Geometry check sheet. Reference: the model listing, model coordinates, mm. A direction names the side the tool comes from. Round coordinates to 2 decimals unless told otherwise and drop trailing zeros. Order: outer loops, then holes, each group sorted by start corner. A loop starts at its lowest first (then second) coordinate and runs counter-clockwise, first axis right, second up. Notation, with made-up numbers: (2.5, 25.5) - (20.5, 25.5) arc R30 ccw to (20.5, 49.5) - close; hole circle Ø6 at (62, 33.5). An arc over 180 degrees is marked (long way). One line per question, with ' | ' between items. Start each with the question number.
Q1. Sectioned sample at C-C, the plane z = 1.5. Enter the section's corners in (x, y).
Q2. Mould release check, pull along Z, two halves, no side actions. Record for faces 1 (the face through (13, 3, 3)), 2 (the face through (14, 4.5, -1)), 3 (the face through (4.24, 2.22, -0.13)): +Z half, -Z half, draft (parallel to the pull), parting line (faces both ways), or undercut.
Q3. Tool access check on faces 4 (the face through (14, 3, -1.2)), 5 (the face through (11, 5, 0)), 6 (the face through (10.272, 4.735, 0.929)), 7 (the face through (11, 1, 0)), 8 (the face through (6.5, 5, 2)). Record the directions out of +Z, -Z, +X, -X, +Y, -Y that give a thin tool (end or side, any length) a straight path to the whole face; none if there is none.
Q4. Material ranges on line 1 along X through (y, z) = (3, 2); line 2 along Z through (x, y) = (-3.25, 1.5); line 3 along X through (y, z) = (2.65, 0), recorded low to high.
Q5. Sectioned sample at D-D, the plane z = -0.5. Enter the section's corners in (x, y), then the cut area to 3 significant figures.
Q6. Sectioned sample at A-A, the plane y = 3. Enter the section's corners in (x, z).
Q7. Gauge pin test, flat ends, axial feed: P1, Ø1, axis at x = 14, z = -1, coming from the +Y side; P2, Ø2.5, axis at x = 13.5, y = 3, coming from the -Z side; P3, Ø1.2, axis at y = 5.5, z = 2, coming from the -X side. Record the tip position at first contact, or that the pin passes through.
Q8. Sectioned sample at B-B, the plane x = 10.5. Enter the section's corners in (y, z).
```python
from build123d import *

# Parameters (mm, degrees)
SKETCH_2_W          = 13
SKETCH_2_H          = 10
SKETCH_2_R          = 1
EXTRUDE_1_DEPTH     = 6
EXTRUDE_3_DEPTH     = 10
SKETCH_5_R          = 1.75
CUT_EXTRUDE_1_DEPTH = 20.293781382
SKETCH_6_W          = 13
SKETCH_6_H          = 10
CUT_EXTRUDE_2_DEPTH = 1.5


with BuildPart() as part:
    # 草图2 → 凸台-拉伸1 (new body)
    with BuildSketch(Plane(origin=(0, 0, 0), x_dir=(1, 0, 0), z_dir=(0, 1, 0))):
        Rectangle(SKETCH_2_W, SKETCH_2_H)
        with Locations(Location((-3.25, 0, 0), (0, 0, 270))):
            Circle(SKETCH_2_R, mode=Mode.SUBTRACT)
        with Locations(Location((3.25, 0, 0), (0, 0, 270))):
            Circle(SKETCH_2_R, mode=Mode.SUBTRACT)
    extrude(amount=EXTRUDE_1_DEPTH)

    # 草图4 → 凸台-拉伸3 (add)
    with BuildSketch(Plane(origin=(6.5, 0, 11.5), x_dir=(0, 0, -1), z_dir=(1, 0, 0))):
        Polygon((11.5, 6), (11.5, 4.5), (12.7, 4.5), (12.7, 1.5), (11.5, 1.5), (11.5, 0), (8.5, 0), (8.5, 6), align=None)
    extrude(amount=EXTRUDE_3_DEPTH)

    # 草图5 → 切除-拉伸1 (cut, through all)
    with BuildSketch(Plane.XY.offset(3)):
        with Locations((10.5, 3)):
            Circle(SKETCH_5_R)
    extrude(amount=-CUT_EXTRUDE_1_DEPTH, mode=Mode.SUBTRACT)

    # 草图6 → 切除-拉伸2 (cut)
    with BuildSketch(Plane(origin=(0, 6, 0), x_dir=(1, 0, 0), z_dir=(0, 1, 0))):
        Rectangle(SKETCH_6_W, SKETCH_6_H)
    extrude(amount=-CUT_EXTRUDE_2_DEPTH, mode=Mode.SUBTRACT)


solid = part.part
```
Determined:
1) outline: (-6.5, 0) - (16.5, 0) - (16.5, 6) - (6.5, 6) - (6.5, 4.5) - (-6.5, 4.5) - close; hole circle Ø3.5 at (10.5, 3)
2) face 1: +Z half | face 2: draft | face 3: undercut
3) face 4: -Z, +X, +Y, -Y | face 5: -Z, +X, -X, +Y | face 6: +Z, -Z | face 7: -Z, +X, -Y | face 8: +Z, -Z, -X, +Y
4) line 1: x = -6.5 to 8.75, 12.25 to 16.5 | line 2: z = -5 to -1, 1 to 5 | line 3: x = -6.5 to -4.25, -2.25 to 2.25, 4.25 to 8.79, 12.21 to 16.5
5) outline: (-6.5, 0) - (-4.12, 0) - (-4.12, 4.5) - (-6.5, 4.5) - close; (-2.38, 0) - (2.38, 0) - (2.38, 4.5) - (-2.38, 4.5) - close; (4.12, 0) - (6.5, 0) - (6.5, 1.5) - (9.6, 1.5) arc R1.75 cw to (9.6, 4.5) - (4.12, 4.5) - close; (11.4, 1.5) - (16.5, 1.5) - (16.5, 4.5) - (11.4, 4.5) arc R1.75 cw to start | area: 63.9 mm2
6) outline: (-6.5, -5) - (6.5, -5) - (6.5, -1.2) - (8.75, -1.2) - (8.75, 3) - (6.5, 3) - (6.5, 5) - (-6.5, 5) - close; (12.25, -1.2) - (16.5, -1.2) - (16.5, 3) - (12.25, 3) - close; hole circle Ø2 at (-3.25, 0); hole circle Ø2 at (3.25, 0)
7) P1: stops at y = 4.5 | P2: stops at z = -1.2 | P3: stops at x = 6.5
8) outline: (0, 0) - (1.25, 0) - (1.25, 3) - (0, 3) - close; (4.75, 0) - (6, 0) - (6, 3) - (4.75, 3) - close
